The model under review builds one solid part; all positions refer to its coordinate system, in mm. Face numbers are marked on the shaded views. A direction names the side the tool comes from. Round coordinates to 2 decimals unless told otherwise and drop trailing zeros. Write each loop counter-clockwise with the first axis right and the second up, starting at its lowest first coordinate (ties: lowest second). Pieces come first, ordered by that corner, then holes. Notation, with made-up numbers: (18, 29) - (72, 29) arc R18 cw to (72, 46) - close; hole circle Ø5 at (-4.75, -13.75). An arc over 180 degrees is marked (long way). One line per question, with ' | ' between items. Start each with the question number.
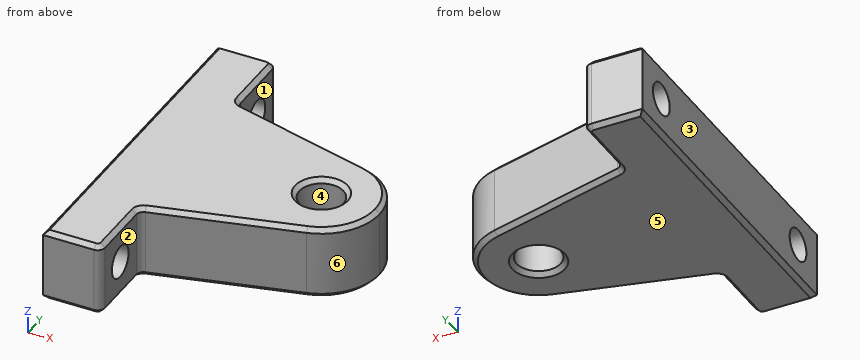
Autodesk Inventor part; units mm, degrees
ref_plane "YZ Plane" through (0, 0, 0) normal (1, 0, 0) x (0, 1, 0)
ref_plane "XZ Plane" through (0, 0, 0) normal (0, 1, 0) x (-1, 0, 0)
ref_plane "XY Plane" through (0, 0, 0) normal (0, 0, 1) x (1, 0, 0)
sketch "Sketch1" plane through (0, 0, 0) normal (0, 0, 1) x (1, 0, 0)
  line L0 (0, 0) -> (0, 11.5)
  line L1 (0, 11.5) -> (4, 11.5)
  line L2 (4, 11.5) -> (4, 6.5)
  line L3 (4, 6.5) -> (14.1296, 3.8718)
  line L4 (-3.5573, 0) -> (21.3437, 0) construction
  circle A0 centre (13.125, 0) radius 1.5125
  arc A1 (17.125, 0) -> (14.1296, 3.8718) centre (13.125, 0) ccw
  line L5 (0, 0) -> (0, -11.5)
  line L6 (0, -11.5) -> (4, -11.5)
  line L7 (4, -11.5) -> (4, -6.5)
  line L8 (4, -6.5) -> (14.1296, -3.8718)
  arc A2 (14.1296, -3.8718) -> (17.125, 0) centre (13.125, 0) ccw
  dimension "d0" = 3.025
  dimension "d1" = 13.125
  dimension "d2" = 4
  dimension "d3" = 11.5
  dimension "d4" = 4
  dimension "d5" = 5
extrude "Extrusion1" add sketch "Sketch1" along normal blind 5
fillet "Fillet1" radius 0.5 4 edges at (4, 6.5, 2.5) (4, -6.5, 2.5) (4, -11.5, 2.5) (4, 11.5, 2.5)
chamfer "Chamfer1" distance 0.3 angle 45 26 edges at (16.2887, 2.4476, 0) (9.252, -5.1373, 0) (4.1045, -6.5809, 0) (4, -8.9434, 0) (3.8536, -11.3536, 0) (1.75, -11.5, 0) (9.252, 5.1373, 0) (4.1045, 6.5809, 0) (4, 8.9434, 0) (3.8536, 11.3536, 0) (1.75, 11.5, 0) (11.6125, 0, 0) (0, 5.75, 0) (4, -8.9434, 5) (4.1045, -6.5809, 5) (9.252, -5.1373, 5) (16.2887, 2.4476, 5) (9.252, 5.1373, 5) (4.1045, 6.5809, 5) (4, 8.9434, 5) (3.8536, 11.3536, 5) (1.75, 11.5, 5) (3.8536, -11.3536, 5) (1.75, -11.5, 5) (11.6125, 0, 5) (0, -5.75, 5)
hole "Hole1" at (4, 9, 2.5) direction (-1, 0, 0) diameter 2.2 end through all
mirror "Mirror1" about plane through (0, 0, 0) normal (0, 1, 0) of "Hole1"
equation "\"d0\" = bore_clearance"
equation "\"d1\" = -0.5 * finger_width + 0.5 * dist_hinge_points"
equation "\"d9\" = champfer"
equation "\"finger_width\" = 25"
equation "\"finger_thickness\" = 8"
equation "\"finger_part_A_length\" = 42.8625"
equation "\"finger_part_B_length\" = 28.575"
equation "\"finger_link_width\" = 3.5"
equation "\"finger_link_clearence\" = 0.075"
equation "\"tol\" = 0.5 * finger_link_clearence"
equation "\"link_tol\" = 0.254"
equation "\"bore_press\" = 2.925"
equation "\"bore_clearance\" = 3.025"
equation "\"bar_diameter\" = 6.5"
equation "\"bar_thickness\" = 4"
equation "\"bar_width\" = 7"
equation "\"hinge_dist_sym_plane\" = 4"
equation "\"hinge_thickness\" = 3"
equation "\"hinge_act_length_c\" = 7.62"
equation "\"hinge_act_length_bc\" = 16.66875"
equation "\"hinge_act_length_ab\" = 11.049"
equation "\"hinge_act_length_a\" = 21.43125"
equation "\"hinge_guid_length_c\" = 9.525"
equation "\"hinge_guid_length_bc\" = 9.525"
equation "\"hinge_guid_length_ab\" = 17.145"
equation "\"hinge_guid_length_a\" = 17.145"
equation "\"bar_length_bc\" = finger_part_B_length"
equation "\"bar_act_length_ab\" = 40.48125"
equation "\"bar_guid_length_ab\" = 43.275"
equation "\"champfer\" = 0.3"
equation "\"fillet\" = 0.4"
equation "\"gear_diameter\" = 14"
equation "\"dist_finger_BC\" = 56.5"
equation "\"hinge_point\" = 15"
properties part number "hinge-axis_mount"
1. Add section B-B, the plane y = -9. Write out the cut boundary in (x, z).
2. Wall thickness on line 1 along Y through (x, z) = (2.25, 2.5); line 2 along Z through (x, y) = (1.45, -9); line 3 along Y through (x, z) = (3.75, 2.7): over which ranges is each line inside the solid? List them lowest first. Write a range as [from, to].
3. Add section D-D, the plane x = 5. Write out the cut boundary in (y, z), then the cut area to 3 significant figures.
4. Clearance check with flat-ended pins moving along their axes: P1, Ø2, axis at y = -9, z = 2.5, coming from the -X side; P2, Ø1.2, axis at y = 9.5, z = 3.5, coming from the +X side. State where each tip first meets the part, or that it passes through.
5. The part is to be moulded in two halves that separate along X. For the marked faces 4, 5 and 6, say which applies: pulls with the +X half, pulls with the -X half, needs draft (parallel to the pull), parting line crosses it, or undercut.
6. Add section C-C, the plane z = 3.9. Write out the cut boundary in (x, y) (1 decimal).
7. Add section A-A, the plane z = 2.5. Write out the cut boundary in (x, y) (1 decimal), then the cut area to 3 significant figures.
8. Machinability: for the marked faces 1, 2 and 3, which of the approach directions +Z, -Z, +X, -X, +Y, -Y give a long, thin tool a straight path to every point of the face, cutting with its end or side? Answer none if there is none.
Geometry check:
1) outline: (0, 0.3) - (0.3, 0) - (3.7, 0) - (4, 0.3) - (4, 1.4) - (0, 1.4) - close; (0, 3.6) - (4, 3.6) - (4, 4.7) - (3.7, 5) - (0.3, 5) - (0, 4.7) - close
2) line 1: y = [-11.5, -10.1], [-7.9, 7.9], [10.1, 11.5] | line 2: z = [0, 1.4], [3.6, 5] | line 3: y = [-11.43, -10.08], [-7.92, 7.92], [10.08, 11.43]
3) outline: (-6.24, 0.3) - (-5.93, 0) - (5.93, 0) - (6.24, 0.3) - (6.24, 4.7) - (5.93, 5) - (-5.93, 5) - (-6.24, 4.7) - close | area: 62.2 mm2
4) P1: passes through | P2: stops at x = 4
5) face 4: undercut | face 5: needs draft | face 6: pulls with the +X half
6) outline: (0, -11.5) - (3.5, -11.5) arc R0.5 ccw to (4, -11) - (4, -6.9) arc R0.5 cw to (4.4, -6.4) - (14.1, -3.9) arc R4 ccw to (17.1, 0) arc R4 ccw to (14.1, 3.9) - (4.4, 6.4) arc R0.5 cw to (4, 6.9) - (4, 11) arc R0.5 ccw to (3.5, 11.5) - (0, 11.5) - close; hole circle Ø3 at (13.1, 0)
7) outline: (0, -11.5) - (3.5, -11.5) arc R0.5 ccw to (4, -11) - (4, -10.1) - (0, -10.1) - close; (0, -7.9) - (4, -7.9) - (4, -6.9) arc R0.5 cw to (4.4, -6.4) - (14.1, -3.9) arc R4 ccw to (17.1, 0) arc R4 ccw to (14.1, 3.9) - (4.4, 6.4) arc R0.5 cw to (4, 6.9) - (4, 7.9) - (0, 7.9) - close; (0, 10.1) - (4, 10.1) - (4, 11) arc R0.5 ccw to (3.5, 11.5) - (0, 11.5) - close; hole circle Ø3 at (13.1, 0) | area: 189 mm2
8) face 1: +Z, -Z, +X, +Y | face 2: +Z, -Z, +X, -Y | face 3: +Z, -Z, -X, +Y, -Y
